Input: part model. Units: mm. Frame: model coordinates. Face numbers are marked on the shaded views. Coordinates: 2 decimals unless noted, no trailing zeros. Write each loop counter-clockwise with the first axis right and the second up, starting at its lowest first coordinate (ties: lowest second). Pieces come first, ordered by that corner, then holes.
1) Section query A-A (y = 0). Output: boundary loops of the cut face in (x, z) (3 decimals), then the cut area to 3 significant figures.
2) Pin query (flat end, axial travel): pin 1 Ø5 at (x, y) = (0, 0) entering from +Z; pin 2 Ø1 at (x, z) = (2.5, 17.5) entering from +Y. Return the tip coordinate at first contact, or that it passes through.
3) Draft query along Y for the marked faces 1, 2 and 3. Return one class per face: pulls with the +Y half, pulls with the -Y half, needs draft (parallel to the pull), parting line crosses it, or undercut.
4) Section query C-C (z = 18.15). Output: boundary loops of the cut face in (x, y) (3 decimals).
5) Line query: L1, parallel to Y at x = 0, z = 17.75 (3 decimals); L2, parallel to X at y = -2.5, z = 17.3; L3, parallel to Y at x = -0.5, z = 17.3. Output: solid intervals per line, ascending.
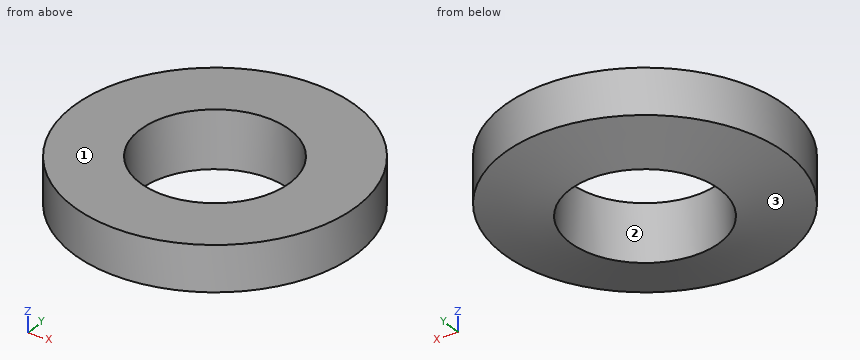
from build123d import *

# Parameters (mm, degrees)
SKETCH043_R     = 6
PAD021_DEPTH    = 3
SKETCH044_R     = 3.175
POCKET021_DEPTH = 3.001


with BuildPart() as part:
    # Sketch043 → Pad021 (new body)
    with BuildSketch(Plane.XY):
        Circle(SKETCH043_R)
    extrude(amount=PAD021_DEPTH)

    # Sketch044 (on Face3 of Pad021) → Pocket021 (cut, through all)
    with BuildSketch(Plane.XY.offset(3)):
        Circle(SKETCH044_R)
    extrude(amount=-POCKET021_DEPTH, mode=Mode.SUBTRACT)

    # Sketch045 → Groove001 (revolve, cut)
    with BuildSketch(Plane.XZ):
        Polygon((0, 0), (12.888196, 2.299908), (13.181708, 0), align=None)
    revolve(axis=Axis((0, 0, 0), (0, 0, 1)), mode=Mode.SUBTRACT)


with BuildPart() as part_1:
    # Body010 placement: moved
    add(part.part.moved(Location((0, 0, 16))))


solid = part_1.part
Answer:
1. outline: (-6, 17.071) - (-3.175, 16.567) - (-3.175, 19) - (-6, 19) - close; (3.175, 16.567) - (6, 17.071) - (6, 19) - (3.175, 19) - close
1. area: 12.3 mm2
2. pin 1: passes through
2. pin 2: stops at y = 5.66
3. face 1: needs draft
3. face 2: undercut
3. face 3: parting line crosses it
4. outline: circle Ø12 at (0, 0); hole circle Ø6.35 at (0, 0)
5. L1: y = -6 to -3.175, 3.175 to 6
5. L2: x = -5.45 to -1.96, 1.96 to 5.45
5. L3: y = -5.98 to -3.14, 3.14 to 5.98
